Autodesk Fusion 360 part; units mm, degrees
sketch "Sketch1" plane through (0, 0, -0.05) normal (0, 0, -1) x (1, 0, 0)
  line L0 (69.1388, 132.6388) -> (69.1388, 72.5424)
  line L1 (69.1388, 72.5424) -> (168.3004, 72.5424)
  line L2 (168.3004, 72.5424) -> (168.3004, 132.6388)
  line L3 (168.3004, 132.6388) -> (69.1388, 132.6388)
  circle A0 centre (75.184, 127.762) radius 1.5875
  circle A1 centre (162.6616, 127.1016) radius 1.5875
  circle A2 centre (105.5624, 117.7544) radius 1.9875
  circle A3 centre (100.4824, 117.7544) radius 0.8374
  circle A4 centre (110.6424, 117.7544) radius 0.8374
  circle A5 centre (101.7524, 115.2144) radius 0.7374
  circle A6 centre (137.5664, 111.8616) radius 1.9875
  circle A7 centre (156.6164, 111.8616) radius 1.9875
  circle A8 centre (108.1024, 112.6744) radius 0.7374
  circle A9 centre (132.4864, 111.8616) radius 0.8374
  circle A10 centre (142.6464, 111.8616) radius 0.8374
  circle A11 centre (151.5364, 111.8616) radius 0.8374
  circle A12 centre (161.6964, 111.8616) radius 0.8374
  circle A13 centre (141.3764, 109.3216) radius 0.7374
  circle A14 centre (160.4264, 109.3216) radius 0.7374
  circle A15 centre (79.5528, 106.9848) radius 1.9875
  circle A16 centre (74.4728, 106.9848) radius 0.8374
  circle A17 centre (84.6328, 106.9848) radius 0.8374
  circle A18 centre (135.0264, 106.7816) radius 0.7374
  circle A19 centre (154.0764, 106.7816) radius 0.7374
  circle A20 centre (75.7428, 104.4448) radius 0.7374
  circle A21 centre (82.0928, 101.9048) radius 0.7374
  circle A22 centre (140.0556, 90.7861) radius 0.4319
  circle A23 centre (155.2956, 90.7861) radius 0.4319
  circle A24 centre (140.0556, 88.2461) radius 0.4319
  circle A25 centre (155.2956, 88.2461) radius 0.4319
  circle A26 centre (101.8032, 85.8012) radius 1.9875
  circle A27 centre (120.8532, 85.8012) radius 1.9875
  circle A28 centre (96.7232, 85.8012) radius 0.8374
  circle A29 centre (106.8832, 85.8012) radius 0.8374
  circle A30 centre (115.7732, 85.8012) radius 0.8374
  circle A31 centre (125.9332, 85.8012) radius 0.8374
  circle A32 centre (140.0556, 85.7061) radius 0.4319
  circle A33 centre (155.2956, 85.7061) radius 0.4319
  circle A34 centre (97.9932, 83.2612) radius 0.7374
  circle A35 centre (117.0432, 83.2612) radius 0.7374
  circle A36 centre (140.0556, 83.1661) radius 0.4319
  circle A37 centre (155.2956, 83.1661) radius 0.4319
  circle A38 centre (104.3432, 80.7212) radius 0.7374
  circle A39 centre (123.3932, 80.7212) radius 0.7374
  circle A40 centre (140.0556, 80.6261) radius 0.4319
  circle A41 centre (155.2956, 80.6261) radius 0.4319
  circle A42 centre (140.0556, 78.0861) radius 0.4319
  circle A43 centre (155.2956, 78.0861) radius 0.4319
  circle A44 centre (79.2988, 76.6064) radius 1.5875
  circle A45 centre (140.0556, 75.5461) radius 0.4319
  circle A46 centre (155.2956, 75.5461) radius 0.4319
  circle A47 centre (75.184, 127.762) radius 1.5875
  circle A48 centre (79.2988, 76.6064) radius 1.5875
  circle A49 centre (162.6616, 127.1016) radius 1.5875
  circle A50 centre (162.6616, 127.1016) radius 3.5
  circle A51 centre (79.2988, 76.6064) radius 3.5
  circle A52 centre (75.184, 127.762) radius 3.5
  dimension "d1" = 7
  dimension "d2" = 7
  dimension "d3" = 7
extrude "Extrude1" add sketch "Sketch1" along normal blind 5 contours A50 | A51 | A52 makes body 1 at (72.8681, -125.1378, -3.3833) makes body 2 at (82.7944, -76.4319, -3.3833) makes body 3 at (165.4516, -129.2149, -3.3833)
sketch "Sketch2" plane through (0, 0, -0.05) normal (0, 0, -1) x (1, 0, 0)
sketch "Sketch3" plane through (0, 0, -5.05) normal (0, 0, -1) x (1, 0, 0)
  circle A0 centre (75.184, 127.762) radius 1.5875
  circle A1 centre (75.184, 127.762) radius 3.5
  line L0 (69.1388, 132.6388) -> (69.1388, 72.5424)
  line L1 (69.1388, 72.5424) -> (168.3004, 72.5424)
  line L2 (168.3004, 72.5424) -> (168.3004, 132.6388)
  line L3 (168.3004, 132.6388) -> (69.1388, 132.6388)
  circle A2 centre (75.184, 127.762) radius 1.5875
  circle A3 centre (162.6616, 127.1016) radius 1.5875
  circle A4 centre (105.5624, 117.7544) radius 1.9875
  circle A5 centre (100.4824, 117.7544) radius 0.8374
  circle A6 centre (110.6424, 117.7544) radius 0.8374
  circle A7 centre (101.7524, 115.2144) radius 0.7374
  circle A8 centre (137.5664, 111.8616) radius 1.9875
  circle A9 centre (156.6164, 111.8616) radius 1.9875
  circle A10 centre (108.1024, 112.6744) radius 0.7374
  circle A11 centre (132.4864, 111.8616) radius 0.8374
  circle A12 centre (142.6464, 111.8616) radius 0.8374
  circle A13 centre (151.5364, 111.8616) radius 0.8374
  circle A14 centre (161.6964, 111.8616) radius 0.8374
  circle A15 centre (141.3764, 109.3216) radius 0.7374
  circle A16 centre (160.4264, 109.3216) radius 0.7374
  circle A17 centre (79.5528, 106.9848) radius 1.9875
  circle A18 centre (74.4728, 106.9848) radius 0.8374
  circle A19 centre (84.6328, 106.9848) radius 0.8374
  circle A20 centre (135.0264, 106.7816) radius 0.7374
  circle A21 centre (154.0764, 106.7816) radius 0.7374
  circle A22 centre (75.7428, 104.4448) radius 0.7374
  circle A23 centre (82.0928, 101.9048) radius 0.7374
  circle A24 centre (140.0556, 90.7861) radius 0.4319
  circle A25 centre (155.2956, 90.7861) radius 0.4319
  circle A26 centre (140.0556, 88.2461) radius 0.4319
  circle A27 centre (155.2956, 88.2461) radius 0.4319
  circle A28 centre (101.8032, 85.8012) radius 1.9875
  circle A29 centre (120.8532, 85.8012) radius 1.9875
  circle A30 centre (96.7232, 85.8012) radius 0.8374
  circle A31 centre (106.8832, 85.8012) radius 0.8374
  circle A32 centre (115.7732, 85.8012) radius 0.8374
  circle A33 centre (125.9332, 85.8012) radius 0.8374
  circle A34 centre (140.0556, 85.7061) radius 0.4319
  circle A35 centre (155.2956, 85.7061) radius 0.4319
  circle A36 centre (97.9932, 83.2612) radius 0.7374
  circle A37 centre (117.0432, 83.2612) radius 0.7374
  circle A38 centre (140.0556, 83.1661) radius 0.4319
  circle A39 centre (155.2956, 83.1661) radius 0.4319
  circle A40 centre (104.3432, 80.7212) radius 0.7374
  circle A41 centre (123.3932, 80.7212) radius 0.7374
  circle A42 centre (140.0556, 80.6261) radius 0.4319
  circle A43 centre (155.2956, 80.6261) radius 0.4319
  circle A44 centre (140.0556, 78.0861) radius 0.4319
  circle A45 centre (155.2956, 78.0861) radius 0.4319
  circle A46 centre (79.2988, 76.6064) radius 1.5875
  circle A47 centre (140.0556, 75.5461) radius 0.4319
  circle A48 centre (155.2956, 75.5461) radius 0.4319
  line L4 (118.7196, 132.6388) -> (118.7196, 72.5424)
  line L5 (118.7196, 102.5906) -> (168.3004, 102.5906)
  line L6 (69.1388, 72.5424) -> (64.8962, 68.2998)
  line L7 (168.3004, 132.6388) -> (172.543, 136.8814)
  line L8 (168.3004, 132.6388) -> (174.3004, 132.6388) construction
  line L9 (64.8962, 68.2998) -> (172.543, 68.2998)
  line L10 (172.543, 68.2998) -> (172.543, 136.8814)
  line L11 (172.543, 136.8814) -> (64.8962, 136.8814)
  line L12 (64.8962, 136.8814) -> (64.8962, 68.2998)
  line L13 (69.1388, 72.5424) -> (168.3004, 72.5424)
  line L14 (168.3004, 72.5424) -> (168.3004, 132.6388)
  line L15 (168.3004, 132.6388) -> (69.1388, 132.6388)
  line L16 (69.1388, 132.6388) -> (69.1388, 72.5424)
  line L17 (139.1248, 68.2998) -> (139.1248, 72.5424)
  line L18 (156.4875, 72.5424) -> (156.4875, 68.2998)
  dimension "d6" = 6
  dimension "d7" = 45
  dimension "d8" = 45
  dimension "d9" = 6
extrude "Extrude2" add sketch "Sketch3" against normal blind 7 separate body contours L0 L3 L6 L7 L11 L12 L15 L16 | L1 L6 L9 L13 L17 | L1 L2 L7 L9 L10 L13 L14 L18 makes body 4
sketch "Sketch4" plane through (0, 0, -5.05) normal (0, 0, -1) x (1, 0, 0)
  line L0 (168.3004, 132.6388) -> (69.1388, 132.6388)
  line L1 (69.1388, 132.6388) -> (69.1388, 72.5424)
  line L2 (69.1388, 72.5424) -> (168.3004, 72.5424)
  line L3 (168.3004, 72.5424) -> (168.3004, 132.6388)
  point P0 (69.1388, 72.5424)
  point P1 (168.3004, 132.6388)
extrude "Extrude3" add sketch "Sketch4" sketch "Sketch3" against normal blind 2 of sketch 2 contours A3 bodies 1 2 3 4
extrude "Extrude4" add sketch "Sketch3" against normal blind 2 contours L1 L9 L13 L17 L18 bodies 1
extrude "Extrude5" cut sketch "Sketch1" along normal mid plane 200 contours A0 A47 | A1 A49 | A44 A48 bodies 1
fillet "Fillet1" radius 2 2 edges at (156.4875, -70.4211, 1.95) (139.1248, -70.4211, 1.95) on bodies 1
fillet "Fillet2" radius 2 4 edges at (172.543, -68.2998, -1.55) (172.543, -136.8814, -1.55) (64.8962, -136.8814, -1.55) (64.8962, -68.2998, -1.55) on bodies 1
extrude "Extrude6" add sketch "Sketch3" against normal blind 5 contours L1 L9 L13 L17 L18 bodies 1
CAD build for the part. Positions are in the model's coordinates, mm. A direction names the side the tool comes from. Round coordinates to 2 decimals unless told otherwise and drop trailing zeros. Loops run counter-clockwise (first coordinate to the right, second up) from the corner with the lowest first, then second, coordinate; pieces in that order, holes last. Notation, with made-up numbers: M -14,68.5 L -7,68.5 A21 cw -7,86.5 Z; hole C 72.5,40 d3. An arc over 180 degrees is marked long. Return JSON: item names as keys, results as strings. Group by question number.
(1) Saw through at B-B, the plane y = -119.5. List the corners of the cut face in (x, z).
(2) Saw through at A-A, the plane z = -1.5. List the corners of the cut face in (x, y) (1 decimal).
(3) Tool access for faces 1 (the cylindrical face through (65.467, -136.28, -1.501)), 2 (the cylindrical face through (138.6, -70.5, 1.3)), 3 (the flat face through (118, -103, -3.05)): list every direction of +Z, -Z, +X, -X, +Y, -Y with a clear straight run to the whole face (end or side of a thin tool).
(4) Mould opens along Y. For faces 4 (the flat face through (119, -136.881, -2)), 5 (the flat face through (64.896, -103, -2)), 6 (the flat face through (119, -132.639, -1)) say: +Y half, -Y half, draft (parallel to the pull), parting line (faces both ways), or undercut.
(5) Wall check: probe 1 along X at (y, z) = (-106.5, -0.75); probe 2 along Y at (x, z) = (167, 1.5); probe 3 along Y at (x, z) = (81.5, -1.75). Give the ranges that are in metal, low to high. Write a range as [from, to].
(6) Saw through at C-C, the plane x = 143. List the corners of the cut face in (y, z), and give its area (3 significant figures).
(7) Drop flat-ended pins along their axis: P1, Ø1.3, axis at x = 151.5, y = -70.5, coming from the +Z side; P2, Ø1, axis at x = 81.5, y = -128, coming from the +Z side. Give the stop position or say it passes through.
Answer list:
{
 "1": {"outline": "M 64.9,-5.05 L 172.54,-5.05 L 172.54,1.95 L 168.3,1.95 L 168.3,-3.05 L 69.14,-3.05 L 69.14,1.95 L 64.9,1.95 Z"},
 "2": {"outline": "M 64.9,-134.9 A2 ccw 66.9,-136.9 L 170.5,-136.9 A2 ccw 172.5,-134.9 L 172.5,-70.3 A2 ccw 170.5,-68.3 L 66.9,-68.3 A2 ccw 64.9,-70.3 Z; C 75.2,-127.8 d7; C 79.3,-76.6 d7; C 162.7,-127.1 d7; hole M 69.1,-132.6 L 168.3,-132.6 L 168.3,-72.5 L 69.1,-72.5 Z; hole C 75.2,-127.8 d3.2; hole C 79.3,-76.6 d3.2; hole C 162.7,-127.1 d3.2"},
 "3": {"face 1": "+Z, -Z, -X, -Y", "face 2": "+Z, +Y", "face 3": "+Z"},
 "4": {"face 4": "-Y half", "face 5": "draft", "face 6": "undercut"},
 "5": {"probe 1": "[64.9, 69.14], [168.3, 172.54]", "probe 2": "[-136.88, -132.64], [-72.54, -68.3]", "probe 3": "[-136.88, -132.64], [-79.33, -73.89], [-72.54, -68.3]"},
 "6": {"outline": "M -136.88,-5.05 L -68.3,-5.05 L -68.3,-0.05 L -72.54,-0.05 L -72.54,-3.05 L -132.64,-3.05 L -132.64,1.95 L -136.88,1.95 Z", "area": "171 mm2"},
 "7": {"P1": "z = -0.05", "P2": "z = -3.05"}
}
